Geometry: final body of the model. Coordinates: model frame, mm. Coordinates: 2 decimals unless noted, no trailing zeros. Write each loop counter-clockwise with the first axis right and the second up, starting at its lowest first coordinate (ties: lowest second). Pieces come first, ordered by that corner, then holes. Notation, with made-up numbers: (47.5, 64.25) - (105.5, 64.25) arc R20 cw to (105.5, 75.25) - close; hole circle Ø5 at (39.25, 75.5). An arc over 180 degrees is marked (long way). Put each result on its own line as item: value.
```python
from build123d import *

# Parameters (mm, degrees)
IZIM1_R                     = 5
IZIM1_R_2                   = 2.5
Y_KSEKLIK_EKSTR_ZYON2_DEPTH = 1
SCALE1_SCALE                = 0.5


with BuildPart() as part:
    # Çizim1 → Yükseklik-Ekstrüzyon2 (new body)
    with BuildSketch(Plane.XY):
        with BuildLine():
            Line((-25, 43.301270189), (-26.146521576, 40.39207739))
            ThreePointArc((-26.146521576, 40.39207739), (-27.544598222, 38.602623821), (-29.691484877, 37.862596744))
            Line((-29.691484877, 37.862596744), (-32.693673826, 37.730024144))
            Line((-32.693673826, 37.730024144), (-33.252115355, 34.777253066))
            ThreePointArc((-33.252115355, 34.777253066), (-34.290118058, 32.757522199), (-36.260310201, 31.628316593))
            Line((-36.260310201, 31.628316593), (-39.184480502, 30.935538106))
            Line((-39.184480502, 30.935538106), (-39.17973637, 27.930427214))
            ThreePointArc((-39.17973637, 27.930427214), (-39.820893366, 25.751969023), (-41.54459596, 24.273587558))
            Line((-41.54459596, 24.273587558), (-44.287157421, 23.045145208))
            Line((-44.287157421, 23.045145208), (-43.719395692, 20.094152054))
            ThreePointArc((-43.719395692, 20.094152054), (-43.940993675, 17.834139505), (-45.357143694, 16.058954583))
            Line((-45.357143694, 16.058954583), (-47.82093971, 14.338366552))
            Line((-47.82093971, 14.338366552), (-46.710273625, 11.546031539))
            ThreePointArc((-46.710273625, 11.546031539), (-46.504462376, 9.284526705), (-47.562892001, 7.275425136))
            Line((-47.562892001, 7.275425136), (-49.660641368, 5.123644113))
            Line((-49.660641368, 5.123644113), (-48.046416828, 2.588887101))
            ThreePointArc((-48.046416828, 2.588887101), (-47.420487313, 0.406004917), (-48.083701146, -1.765839874))
            Line((-48.083701146, -1.765839874), (-49.741090048, -4.272585973))
            Line((-49.741090048, -4.272585973), (-47.680491761, -6.459969953))
            ThreePointArc((-47.680491761, -6.459969953), (-46.656617846, -8.486899797), (-46.901121207, -10.744549126))
            Line((-46.901121207, -10.744549126), (-48.059435816, -13.517457571))
            Line((-48.059435816, -13.517457571), (-45.625461503, -15.279979352))
            ThreePointArc((-45.625461503, -15.279979352), (-44.239914432, -17.079151855), (-44.057045667, -19.342627369))
            Line((-44.057045667, -19.342627369), (-44.675252109, -22.283466496))
            Line((-44.675252109, -22.283466496), (-41.954126526, -23.558687864))
            ThreePointArc((-41.954126526, -23.558687864), (-40.255989993, -25.066366444), (-39.652227319, -27.255483394))
            Line((-39.652227319, -27.255483394), (-39.708425324, -30.260072511))
            Line((-39.708425324, -30.260072511), (-36.7965457, -31.002818113))
            ThreePointArc((-36.7965457, -31.002818113), (-34.84597704, -32.165592505), (-33.842709051, -34.202800331))
            Line((-33.842709051, -34.202800331), (-33.334907776, -37.164700371))
            Line((-33.334907776, -37.164700371), (-30.335428898, -37.348658075))
            ThreePointArc((-30.335428898, -37.348658075), (-28.201527977, -38.125336415), (-26.834295942, -39.938466016))
            Line((-26.834295942, -39.938466016), (-25.73775467, -42.866863479))
            ThreePointArc((-25.73775467, -42.866863479), (-24.554196145, -43.55561332), (-23.352220135, -44.21169319))
            ThreePointArc((-23.352220135, -44.21169319), (-17.219408632, -49.939828574), (-14.829333353, -57.984109281))
            ThreePointArc((-14.829333353, -57.984109281), (-20.099106379, -76.543069457), (-25, -57.883306535))
            Line((-25, -57.883306535), (-25, -57.052607302))
            ThreePointArc((-25, -57.052607302), (-25.590454576, -54.960957236), (-27.1875, -53.486819346))
            ThreePointArc((-27.1875, -53.486819346), (-59.999999835, 0.004450967), (-27.179564099, 53.490852446))
            ThreePointArc((-27.179564099, 53.490852446), (-24.232021318, 53.76021953), (-21.906244367, 51.929556087))
            ThreePointArc((-21.906244367, 51.929556087), (-21.212806241, 47.755648425), (-23.446136356, 44.161959762))
            ThreePointArc((-23.446136356, 44.161959762), (-24.226890609, 43.73851588), (-25, 43.301270189))
        make_face()
        with Locations((-20, -66.543560573)):
            Circle(IZIM1_R, mode=Mode.SUBTRACT)
        with Locations((-31.620079453, -45.001895242)):
            Circle(IZIM1_R_2, mode=Mode.SUBTRACT)
        with Locations((-55, 0)):
            Circle(IZIM1_R_2, mode=Mode.SUBTRACT)
        with Locations((-28.000624989, 47.338831842)):
            Circle(IZIM1_R_2, mode=Mode.SUBTRACT)
    extrude(amount=Y_KSEKLIK_EKSTR_ZYON2_DEPTH)


with BuildPart() as part_1:
    # Scale1: scaled about (-39.321045235, -11.426802876, 0.5)
    add(part.part.scale(SCALE1_SCALE).moved(Location((-19.660522617, -5.713401438, 0.25))))


solid = part_1.part
```
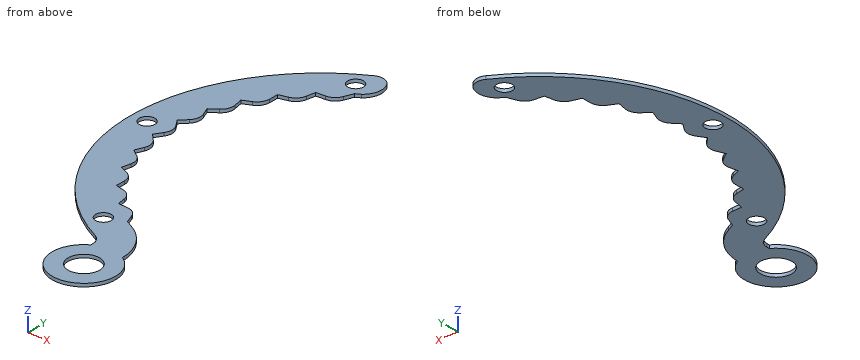
1. Ray query, probe 1 along Y at (x, z) = (-44, 0.7); probe 2 along X at (y, z) = (-40, 0.45); probe 3 along Y at (x, z) = (-46.75, 0.3). Return the intervals inside material, ascending. Write a range as from..to.
Answer below:
probe 1: y = -23.25..-8.41, -7.05..-3.92, -2.65..11.82
probe 2: x = -34.56..-31.95, -27.38..-24.76
probe 3: y = -18.6..-6.89, -4.53..7.18
2. Section query C-C (y = -20). Return loops of the section in (x, z), then the cut area to 3 significant figures.
Answer below:
outline: (-46.04, 0.25) - (-39.5, 0.25) - (-39.5, 0.75) - (-46.04, 0.75) - close
area: 3.27 mm²
3. Section query A-A (x = -47). Return loops of the section in (y, z), then the cut area to 3 significant figures.
Answer below:
outline: (-18.06, 0.25) - (-6.95, 0.25) - (-6.95, 0.75) - (-18.06, 0.75) - close; (-4.47, 0.25) - (6.64, 0.25) - (6.64, 0.75) - (-4.47, 0.75) - close
area: 11.1 mm²
4. Section query B-B (z = 0.5). Count the separate pieces of the cut face and the enclosed holes in it, then the cut area to 3 significant figures.
Answer below:
separate pieces: 1
enclosed holes: 4
area: 420 mm²
5. Section query D-D (y = 7). Return loops of the section in (x, z).
Answer below:
outline: (-46.83, 0.25) - (-39.69, 0.25) - (-39.69, 0.75) - (-46.83, 0.75) - close
6. Pin query (flat end, axial travel): pin 1 Ø8 at (x, y) = (-33.5, -21.5) entering from +Z; pin 2 Ø5 at (x, y) = (-40, -8.5) entering from -Z. Return the tip coordinate at first contact, or that it passes through.
Answer below:
pin 1: stops at z = 0.75
pin 2: passes through
